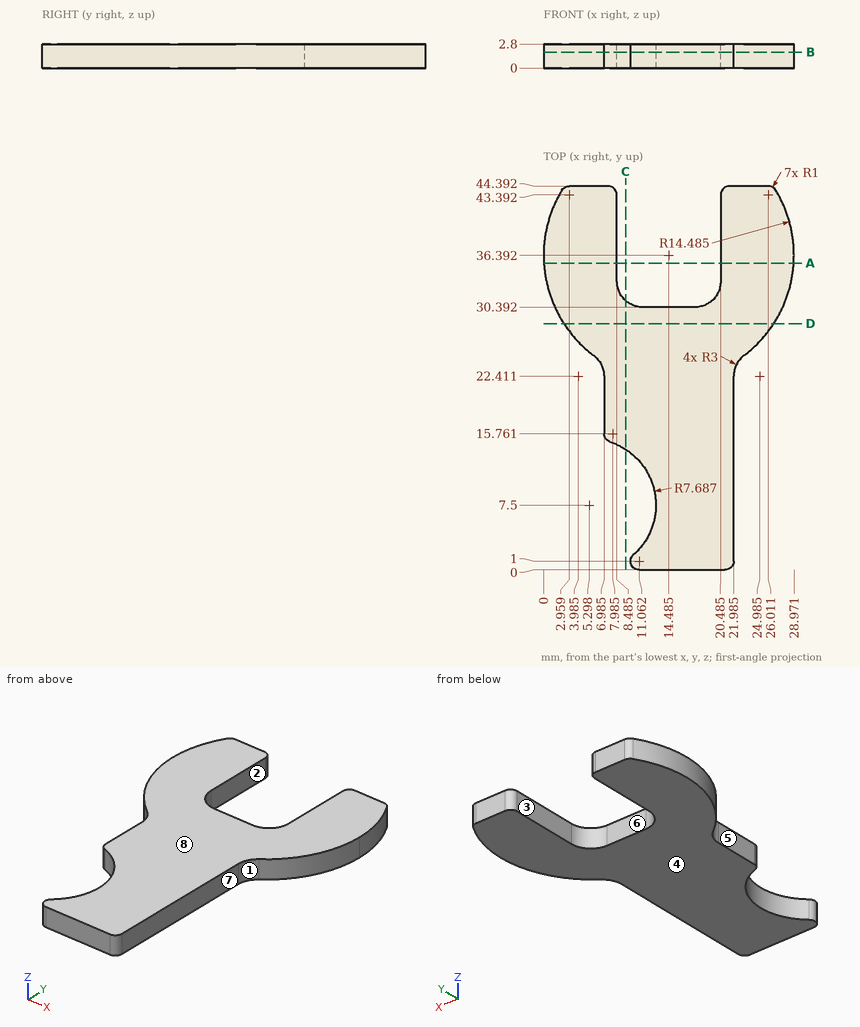
Can you work these out from the drawing? Everything is in mm from the part's minimum corner. A direction names the side the tool comes from. Round coordinates to 2 decimals unless told otherwise and drop trailing zeros. Write each loop counter-clockwise with the first axis right and the second up, starting at its lowest first coordinate (ties: lowest second). Pieces come first, ordered by that corner, then holes.
1. If we mould it in two halves opening along X, with no side actions, what happens to the marked faces 1, 2, 3 and 4? For each: released by +X, released by -X, zero draft, split by the parting line, or undercut.
2. I need wall thicknesses on L1, parallel to X at y = 14.5, z = 2.2 (1 decimal); L2, parallel to Y at x = 16, z = 0.15; L3, parallel to X at y = 34, z = 1.65 (1 decimal). Which ranges of each line are inside material? Lowest first, please.
3. Suppose I cut it at D-D (y = 28.5). List the corners of the cut face in (x, z) for me.
4. Suppose I cut it at C-C (x = 9.5). List the corners of the cut face in (y, z) for me.
5. For the marked faces 5, 6, 7 and 8, which set-ups out of +Z, -Z, +X, -X, +Y, -Y let a thin tool reach every point of the face, with its end or its side?
6. Will these pins go through, and if not, where does the flat tip stop? pin 1 Ø1.4 at (y, z) = (10.5, 1) entering from +X (1 decimal); pin 2 Ø2 at (x, y) = (19, 36) entering from -Z; pin 3 Ø0.8 at (x, z) = (13.5, 2) entering from +Y.
7. Suppose I cut it at A-A (y = 35.5). List the corners of the cut face in (x, z) for me (1 decimal).
8. Suppose I cut it at B-B (z = 1.85). List the corners of the cut face in (x, y) for me (1 decimal), and give its area (3 significant figures).
Answer sheet:
1. face 1: released by +X
1. face 2: undercut
1. face 3: undercut
1. face 4: zero draft
2. L1: x = 8.5 to 22
2. L2: y = 0 to 30.39
2. L3: x = 0.2 to 8.5, 20.5 to 28.8
3. outline: (2.34, 0) - (26.63, 0) - (26.63, 2.8) - (2.34, 2.8) - close
4. outline: (13.94, 0) - (31.14, 0) - (31.14, 2.8) - (13.94, 2.8) - close
5. face 5: +Z, -Z, -X, -Y
5. face 6: +Z, -Z, +Y
5. face 7: +Z, -Z, +X, -Y
5. face 8: +Z, +X, -X, +Y, -Y
6. pin 1: stops at x = 22
6. pin 2: passes through
6. pin 3: stops at y = 30.39
7. outline: (0, 0) - (8.5, 0) - (8.5, 2.8) - (0, 2.8) - close; (20.5, 0) - (28.9, 0) - (28.9, 2.8) - (20.5, 2.8) - close
8. outline: (2.1, 43.9) arc R14.5 ccw to (5.8, 24.8) arc R3 cw to (7, 22.4) - (7, 15.8) arc R1 ccw to (7.7, 14.8) arc R7.7 cw to (10.4, 1.7) arc R1 ccw to (11.1, 0) - (21, 0) arc R1 ccw to (22, 1) - (22, 22.4) arc R3 cw to (23.2, 24.8) arc R14.5 ccw to (26.9, 43.9) arc R1 ccw to (26, 44.4) - (21.5, 44.4) arc R1 ccw to (20.5, 43.4) - (20.5, 33.4) arc R3 cw to (17.5, 30.4) - (11.5, 30.4) arc R3 cw to (8.5, 33.4) - (8.5, 43.4) arc R1 ccw to (7.5, 44.4) - (3, 44.4) arc R1 ccw to start
8. area: 654 mm2
